Geometry: see drawing. Coordinates: mm, zero at the bounding-box minimum. Give positions to 0.01 mm unless a question says otherwise; leave off trailing zeros. Order: outer loops, then holes, each group sorted by start corner. A loop starts at its lowest first (then second) coordinate and runs counter-clockwise, first axis right, second up. Notation, with made-up numbers: M -35.5,30.25 L 16.5,30.25 A31 cw 16.5,57.25 Z; hole C -4,26.5 d9. An arc over 180 degrees is marked long. Answer as a JSON object with one key per item and string values. Group by question number.
1. Section query D-D (y = 53). Output: boundary loops of the cut face in (x, z).
2. Section query A-A (x = 34). Output: boundary loops of the cut face in (y, z).
3. Section query C-C (y = 39). Output: boundary loops of the cut face in (x, z).
4. Material intervals for L1, parallel to Y at x = 27, z = 1.5; L2, parallel to Y at x = 30, z = 1; L3, parallel to X at y = 27, z = 0.35, sorted ascending. Write a range as [from, to].
5. Pin query (flat end, axial travel): P1, Ø1, axis at x = 1, z = 0.5, coming from the +Y side; P2, Ø1, axis at x = 54, z = 0.5, coming from the +Y side; P3, Ø0.6, axis at y = 11.5, z = 1, coming from the -X side. Return the tip coordinate at first contact, or that it passes through.
6. Section query B-B (z = 0.65). Output: boundary loops of the cut face in (x, y).
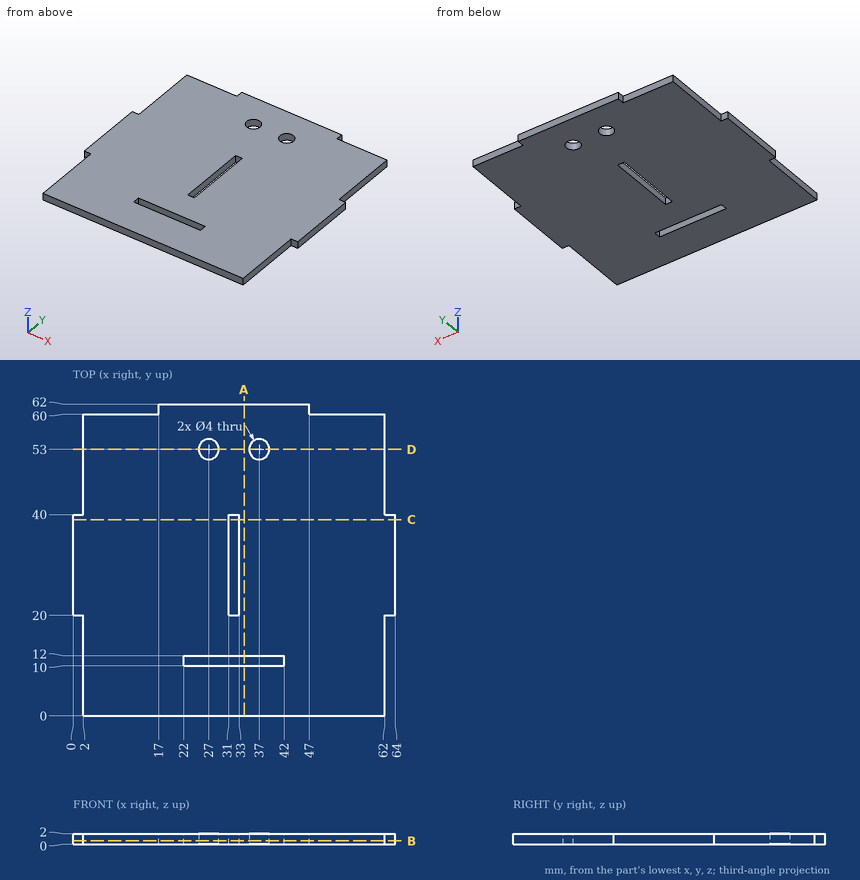
Answer sheet:
{
 "1": {"outline": "M 2,0 L 25,0 L 25,2 L 2,2 Z; M 29,0 L 35,0 L 35,2 L 29,2 Z; M 39,0 L 62,0 L 62,2 L 39,2 Z"},
 "2": {"outline": "M 0,0 L 10,0 L 10,2 L 0,2 Z; M 12,0 L 62,0 L 62,2 L 12,2 Z"},
 "3": {"outline": "M 0,0 L 31,0 L 31,2 L 0,2 Z; M 33,0 L 64,0 L 64,2 L 33,2 Z"},
 "4": {"L1": "[0, 10], [12, 51], [55, 62]", "L2": "[0, 10], [12, 62]", "L3": "[0, 31], [33, 64]"},
 "5": {"P1": "y = 40", "P2": "y = 60", "P3": "x = 2"},
 "6": {"outline": "M 0,20 L 2,20 L 2,0 L 62,0 L 62,20 L 64,20 L 64,40 L 62,40 L 62,60 L 47,60 L 47,62 L 17,62 L 17,60 L 2,60 L 2,40 L 0,40 Z; hole M 22,10 L 42,10 L 42,12 L 22,12 Z; hole C 27,53 d4; hole M 31,20 L 33,20 L 33,40 L 31,40 Z; hole C 37,53 d4"}
}
